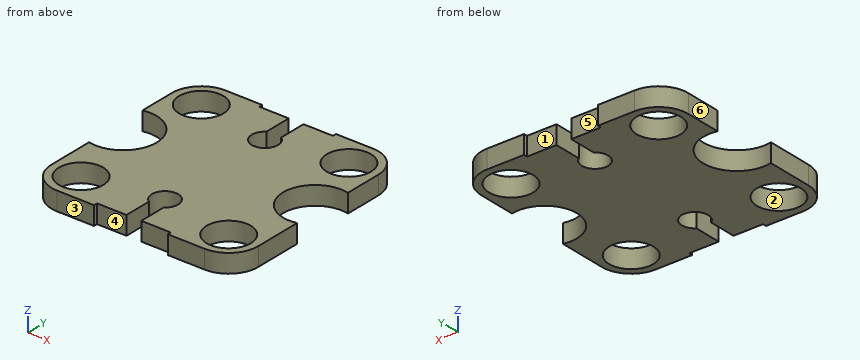
Autodesk Fusion 360 part; units mm, degrees
sketch "Sketch1" plane through (0, 0, 0) normal (0, 0, 1) x (1, 0, 0)
  circle A0 centre (-55.475, -25) radius 30
  circle A1 centre (144.525, -25) radius 30
  circle A2 centre (144.525, -225) radius 30
  circle A3 centre (-55.475, -225) radius 30
  line L0 (-55.475, 15) -> (144.525, 15)
  line L1 (144.525, -265) -> (-55.475, -265)
  line L2 (-95.475, 15) -> (184.525, -265) construction
  line L3 (184.525, 15) -> (-95.475, -265) construction
  line L4 (184.525, -25) -> (184.525, -75.8302)
  line L5 (184.525, -160.367) -> (184.525, -225)
  arc A4 (184.525, -75.8302) -> (184.525, -160.367) centre (174.525, -118.0986) ccw
  line L6 (-95.475, -225) -> (-95.475, -162.4976)
  line L7 (-95.475, -73.6997) -> (-95.475, -25)
  arc A5 (-95.475, -162.4976) -> (-95.475, -73.6997) centre (-85.475, -118.0986) ccw
  arc A6 (-55.475, 15) -> (-95.475, -25) centre (-55.475, -25) ccw
  arc A7 (184.525, -25) -> (144.525, 15) centre (144.525, -25) ccw
  arc A8 (144.525, -265) -> (184.525, -225) centre (144.525, -225) ccw
  arc A9 (-95.475, -225) -> (-55.475, -265) centre (-55.475, -225) ccw
  line L8 (-5.475, -265) -> (-5.475, -260)
  line L9 (94.525, -265) -> (94.525, -260)
  line L10 (-5.475, -260) -> (34.525, -260)
  line L11 (94.525, -260) -> (54.525, -260)
  line L12 (34.525, -260) -> (34.525, -222.8224)
  line L13 (54.525, -260) -> (54.525, -222.8224)
  arc A10 (54.525, -222.8224) -> (34.525, -222.8224) centre (44.525, -208.0986) ccw
  line L14 (34.525, 10) -> (34.525, -27.1776)
  arc A11 (34.525, -27.1776) -> (54.525, -27.1776) centre (44.525, -41.9014) ccw
  line L15 (54.525, 10) -> (54.525, -27.1776)
  line L16 (-5.475, 10) -> (34.525, 10)
  line L17 (94.525, 10) -> (54.525, 10)
  line L18 (-5.475, 15) -> (-5.475, 10)
  line L19 (94.525, 15) -> (94.525, 10)
  point P0 (44.525, -125)
  dimension "d1" = 60
  dimension "d2" = 60
  dimension "d3" = 200
  dimension "d4" = 200
  dimension "d5" = 200
  dimension "d8" = 260
  dimension "d9" = 280
  dimension "d10" = 280
  dimension "d11" = 40
  dimension "d12" = 40
  dimension "d13" = 40
  dimension "d14" = 40
  dimension "d15" = 40
  dimension "d16" = 40
  dimension "d17" = 40
  dimension "d18" = 100
  dimension "d19" = 50
  dimension "d20" = 5
  dimension "d21" = 5
  dimension "d22" = 40
  dimension "d23" = 40
extrude "Extrude1" add sketch "Sketch1" along normal blind 25 contours L0 L1 L4 L5 A4 L6 L7 A5 A6 A7 A8 A9 L8 L9 L10 L11 L12 L13 A10 L14 A11 L15 L16 L17 L18 L19
The listing builds one solid part. Answer for the finished solid, in the listing's coordinates (mm). Face numbers are marked on the shaded views. A direction names the side the tool comes from. Give positions to 0.01 mm unless a question says otherwise; leave off trailing zeros. Order: outer loops, then holes, each group sorted by start corner. A loop starts at its lowest first (then second) coordinate and runs counter-clockwise, first axis right, second up. Notation, with made-up numbers: M -14,87 L 40,87 A9 ccw 40,103 Z; hole C 76,37.25 d10. An arc over 180 degrees is marked long. Put each result on its own line as item: value. Start each with the question number.
Item 1: Flat-ended cylindrical pins translate along their axes: P1, Ø2.5, axis at y = -262, z = 17, coming from the +X side; P2, Ø12.5, axis at x = 70.5, z = 17, coming from the +Y side; P3, Ø12.5, axis at y = -9, z = 10.5, coming from the -X side; P4, Ø21.5, axis at x = 44.52, y = -41.9, coming from the +Z side. Find the tip coordinate at first contact, or state that the pin passes through.
Item 2: Which of the six approach directions +Z, -Z, +X, -X, +Y, -Y give full straight-line access (tool end or side, diameter ignored) to the marked faces 4, 5 and 6?
Item 3: Find the intervals of material crossed by line 1 along Y through (x, z) = (-79.5, 2.5); line 2 along Y through (x, z) = (143, 10.5); line 3 along X through (y, z) = (-249, 9.25) (3 decimals), in increasing order.
Item 4: The part is cut by section B-B, the plane y = -100.5. Determine the outline of the cut face in (x, z).
Item 5: For a pull along Y with two mould halves and no side action, classify the marked faces 1, 2 and 3 as +Y half, -Y half, draft (parallel to the pull), parting line (faces both ways), or undercut.
Item 6: The part is cut by section A-A, the plane z = 12.25. State how many separate pieces and enclosed holes the cut face has, and give its area (3 significant figures).
Answer key:
1. P1: stops at x = 162.47
1. P2: stops at y = 10
1. P3: stops at x = -94.27
1. P4: passes through
2. face 4: +Z, -Z, -Y
2. face 5: +Z, -Z, +Y
2. face 6: +Z, -Z, -X, +Y, -Y
3. line 1: y = -256.98 to -242.97, -207.03 to -163.22, -72.98 to -42.97, -7.03 to 6.98
3. line 2: y = -265 to -254.96, -195.04 to -147.98, -88.22 to -54.96, 4.96 to 15
3. line 3: x = -87.475 to -73.475, -37.475 to 34.525, 54.525 to 126.525, 162.525 to 176.525
4. outline: M -43.5,0 L 134.81,0 L 134.81,25 L -43.5,25 Z
5. face 1: +Y half
5. face 2: undercut
5. face 3: -Y half
6. separate pieces: 1
6. enclosed holes: 4
6. area: 53,300 mm²
